from build123d import *

# Parameters (mm, degrees)
BOSS_EXTRUDE1_DEPTH      = 4
BOSS_EXTRUDE1_DEPTH_BACK = 4
SHELL1_T                 = -1
CUT_EXTRUDE1_DEPTH       = 33.543240466
CUT_EXTRUDE1_DEPTH_BACK  = 33.543240466
SKETCH2_R                = 1
CUT_EXTRUDE2_REACH       = 35.779
CUT_EXTRUDE2_END_RADIUS  = 14
SKETCH3_W                = 2.5
SKETCH3_H                = 1.5
FILLET2_R                = 1


with BuildPart() as part:
    # Sketch1 → Boss-Extrude1 (new, two sides: drawn at the far end of the back side and taken through both)
    with BuildSketch(Plane.XY.offset(-BOSS_EXTRUDE1_DEPTH_BACK)):
        with BuildLine():
            Line((-2.25, -2), (27.75, -2))
            Line((27.75, -2), (27.75, 0))
            ThreePointArc((27.75, 0), (12.75, 15), (-2.25, 0))
            Line((-2.25, 0), (-2.25, -2))
        make_face()
    extrude(amount=BOSS_EXTRUDE1_DEPTH + BOSS_EXTRUDE1_DEPTH_BACK)

    # Shell1
    shell1_openings = [part.faces().sort_by_distance(p)[0] for p in [
        (12.75, -2, 0),
    ]]
    offset(amount=SHELL1_T, openings=shell1_openings, kind=Kind.INTERSECTION)

    # Sketch2 → Cut-Extrude1 (cut, two sides: drawn at the far end of the back side and taken through both)
    with BuildSketch(Plane.XY.offset(4).offset(-CUT_EXTRUDE1_DEPTH_BACK)):
        with Locations(Location((0, 0, 0), (0, 0, 180))):
            Circle(SKETCH2_R)
    extrude(amount=CUT_EXTRUDE1_DEPTH + CUT_EXTRUDE1_DEPTH_BACK, mode=Mode.SUBTRACT)

    # Cut-Extrude2: up to this cylinder (the profile starts outside it)
    cut_extrude2_end = Plane(origin=(12.75, 0, 0), z_dir=(0, 0, 1)) * Cylinder(CUT_EXTRUDE2_END_RADIUS, 100.558, mode=Mode.PRIVATE)
    # Sketch3 → Cut-Extrude2 (cut, up to the surface)
    with BuildSketch(Plane(origin=(27.75, 0, 0), x_dir=(0, 0, -1), z_dir=(1, 0, 0)), mode=Mode.PRIVATE) as cut_extrude2_sk1:
        with Locations((0, -0.25)):
            Rectangle(SKETCH3_W, SKETCH3_H)
    cut_extrude2_tool1 = extrude(cut_extrude2_sk1.sketch, amount=-CUT_EXTRUDE2_REACH, mode=Mode.PRIVATE) - cut_extrude2_end
    add(cut_extrude2_tool1.solids().sort_by_distance((27.75, -0.25, 0))[0], mode=Mode.SUBTRACT)

    # Fillet2
    fillet2_edges = [part.edges().sort_by_distance(p)[0] for p in [
        (27.75, -2, 0),
        (-2.25, -2, 0),
    ]]
    fillet(fillet2_edges, radius=FILLET2_R - 0.0001)  # a hair under: the kernel refuses the full size


solid = part.part
Source: CAD feature listing. Evaluate the final solid. Frame: model axes, mm. A direction names the side the tool comes from. Give positions to 0.01 mm unless a question says otherwise; leave off trailing zeros. Order: outer loops, then holes, each group sorted by start corner. A loop starts at its lowest first (then second) coordinate and runs counter-clockwise, first axis right, second up. Notation, with made-up numbers: (22.25, 15.25) -> (65.25, 15.25) arc R17 ccw to (65.25, 37.25) -> close; hole circle Ø5 at (42.25, 51). An arc over 180 degrees is marked (long way). Use a Markdown table: item, result.
1) Section query D-D, the plane x = 0. Return the cut outline in (y, z), then the cut area to 3 significant figures.
Answer list:
| item | result |
|---|---|
| outline | (-2, -4) -> (-1, -4) -> (-1, -3) -> (-2, -3) -> close; (-2, 3) -> (-1, 3) -> (-1, 4) -> (-2, 4) -> close; (1, -4) -> (7.9, -4) -> (7.9, 4) -> (1, 4) -> (1, 3) -> (5.78, 3) -> (5.78, -3) -> (1, -3) -> close |
| area | 28.5 mm² |
2) Mould query, pull axis Y, two halves, no side actions, for faces 4 (the flat face through (27, 0, 1.25)), 5 (the cylindrical face through (13.058, 13.997, -0.042)), 6 (the cylindrical face through (0.217, 0.976, 3.493)), 7 (the flat face through (13, 4, 3)). Classes: +Y half, -Y half, draft (parallel to the pull), parting line (faces both ways), or undercut.
Answer list:
| item | result |
|---|---|
| face 4 | undercut |
| face 5 | -Y half |
| face 6 | undercut |
| face 7 | draft |
3) Reachability of faces 1 (the flat face through (27, 0.5, 0)), 2 (the flat face through (13, 5, 4)), 3 (the flat face through (-1.25, -1, 0)) from +Z, -Z, +X, -X, +Y, -Y: full face, straight path, thin tool, end or side. Return the list, or none.
Answer list:
| item | result |
|---|---|
| face 1 | +X |
| face 2 | +Z, +X, -X, +Y, -Y |
| face 3 | -Y |
4) Ray query, line 1 along X through (y, z) = (-1, 1.75); line 2 along Z through (x, y) = (23.5, 2.5); line 3 along Y through (x, z) = (0, 3.7). Return the intervals inside material, ascending. Write a range as [from, to].
Answer list:
| item | result |
|---|---|
| line 1 | [-2.25, -1.25], [26.75, 27.75] |
| line 2 | [-4, -3], [3, 4] |
| line 3 | [-2, -1], [1, 7.9] |
5) Section query B-B, the plane x = 12.75. Return the cut outline in (y, z), then the cut area to 3 significant figures.
Answer list:
| item | result |
|---|---|
| outline | (-2, -4) -> (15, -4) -> (15, 4) -> (-2, 4) -> (-2, 3) -> (14, 3) -> (14, -3) -> (-2, -3) -> close |
| area | 40.0 mm² |
6) Section query C-C, the plane y = 8.25. Return the cut outline in (x, z), then the cut area to 3 significant figures.
Answer list:
| item | result |
|---|---|
| outline | (0.22, -4) -> (25.28, -4) -> (25.28, 4) -> (0.22, 4) -> close; hole (1.44, -3) -> (24.06, -3) -> (24.06, 3) -> (1.44, 3) -> close |
| area | 64.7 mm² |
7) Contact query for a flat-ended pin moving along its axis: P1, Ø1, axis at x = 3, z = 2, coming from the +Y side. Output: stop coordinate, or through.
Answer list:
| item | result |
|---|---|
| P1 | y = 11.81 |
